Verification items for this drawing (mm, ordinates from the low corner). A direction names the side the tool comes from. Coordinates: 2 decimals unless noted, no trailing zeros. Order: outer loops, then holes, each group sorted by start corner. A loop starts at its lowest first (then second) coordinate and runs counter-clockwise, first axis right, second up. Notation, with made-up numbers: (75.5, 65.5) - (100.5, 65.5) arc R20 cw to (100.5, 80.5) - close; hole circle Ø3 at (-15, -25.75). An arc over 180 degrees is marked (long way). Use CSV: the item, a comma, the result in double quotes. Start each with the question number.
1) Sectioned sample at D-D, the plane x = 0.5. Record the cut outline in (y, z) (1 decimal).
2) Tool access check on the marked faces 1, 2 and 3. Record the directions out of +Z, -Z, +X, -X, +Y, -Y that give a thin tool (end or side, any length) a straight path to the whole face; none if there is none.
3) Depth check by flat-ended pin: P1, Ø1, axis at x = 2.5, z = 1.5, coming from the -Y side. Enter the tip coordinate at first touch or a pass-through.
4) Sectioned sample at C-C, the plane z = 4.1. Record the cut outline in (x, y).
5) Thickness scan on probe 1 along Z at (x, y) = (2.75, 19.3) (1 decimal); probe 2 along Y at (x, z) = (4.6, 3.65); probe 3 along X at (y, z) = (14.5, 2.25) (1 decimal). Record the ranges inside material, lowest first. Write a range as [from, to].
6) Sectioned sample at B-B, the plane y = 13.5. Record the cut outline in (x, z) (1 decimal).
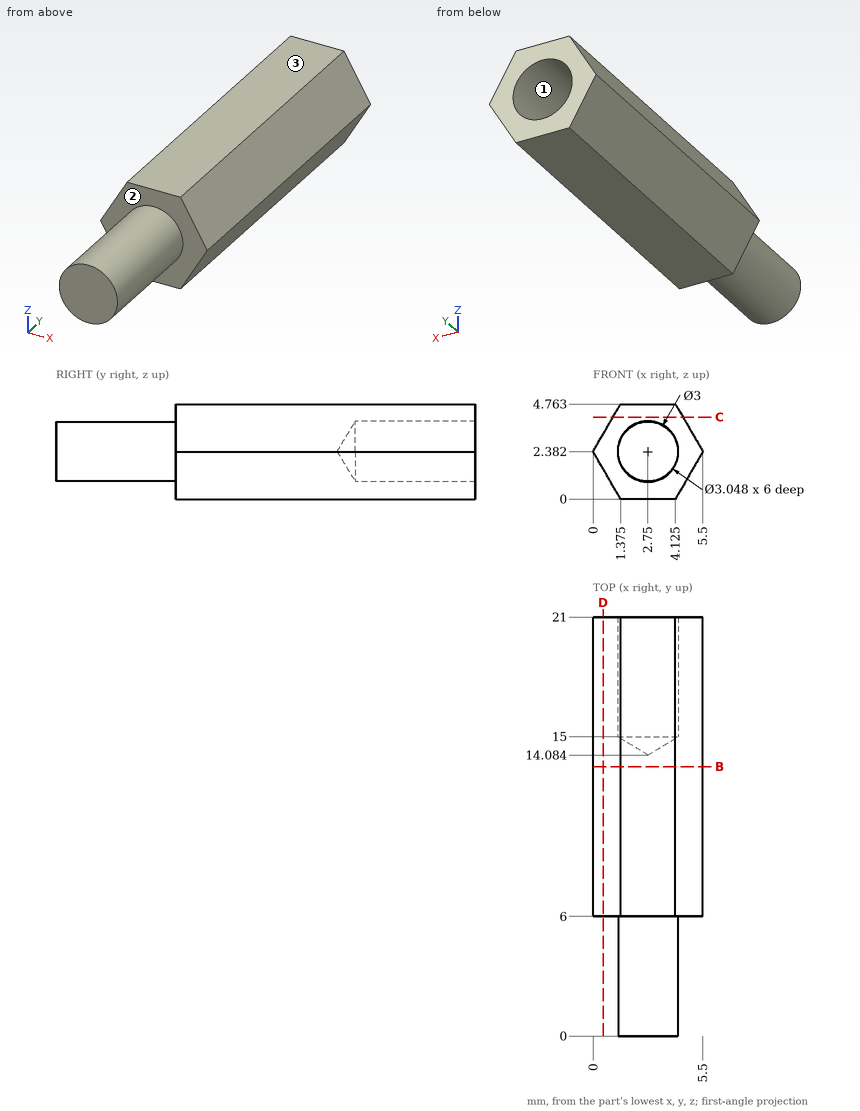
Evaluation:
1,outline,"(6, 1.5) - (21, 1.5) - (21, 3.2) - (6, 3.2) - close"
2,face 1,"+Y"
2,face 2,"-Y"
2,face 3,"+Z, +X, -X, +Y, -Y"
3,P1,"y = 0"
4,outline,"(0.99, 6) - (4.51, 6) - (4.51, 21) - (0.99, 21) - close"
5,probe 1,"[0, 0.9], [3.9, 4.8]"
5,probe 2,"[6, 21]"
5,probe 3,"[0.1, 2.1], [3.4, 5.4]"
6,outline,"(0, 2.4) - (1.4, 0) - (4.1, 0) - (5.5, 2.4) - (4.1, 4.8) - (1.4, 4.8) - close"
